CAD build for the part. Positions are in the model's coordinates, mm. Give positions to 0.01 mm unless a question says otherwise; leave off trailing zeros. Order: outer loops, then holes, each group sorted by start corner. A loop starts at its lowest first (then second) coordinate and runs counter-clockwise, first axis right, second up.
```python
from build123d import *

# Parameters (mm, degrees)
SKETCH1_5_R         = 2.5
BOSS_EXTRUDE4_DEPTH = 3


with BuildPart() as part:
    # Sketch1_5 → Boss-Extrude4 (new body)
    # profile 1 of 2: a face of its own
    with BuildSketch(Plane(origin=(0, 0, 0), x_dir=(1, 0, 0), z_dir=(0, 1, 0))):
        Polygon((0, 25.4), (0, 0), (15, 0), (197, 0), (212, 0), (212, 25.4), align=None)
        with Locations(Location((75.666666667, 12.7, 0), (0, 0, 270))):
            Circle(SKETCH1_5_R, mode=Mode.SUBTRACT)
        with Locations(Location((136.333333333, 12.7, 0), (0, 0, 270))):
            Circle(SKETCH1_5_R, mode=Mode.SUBTRACT)
    # profile 2 of 2: a face of its own
    with BuildSketch(Plane(origin=(0, 0, 0), x_dir=(1, 0, 0), z_dir=(0, 1, 0))):
        Polygon((0, -93), (0, 0), (15, 0), (15, -78), (197, -78), (197, 0), (212, 0), (212, -93), align=None)
        with Locations(Location((136.333333333, -85.5, 0), (0, 0, 270))):
            Circle(SKETCH1_5_R, mode=Mode.SUBTRACT)
        with Locations(Location((75.666666667, -85.5, 0), (0, 0, 270))):
            Circle(SKETCH1_5_R, mode=Mode.SUBTRACT)
        with Locations(Location((204.5, -39, 0), (0, 0, 270))):
            Circle(SKETCH1_5_R, mode=Mode.SUBTRACT)
        with Locations(Location((7.5, -39, 0), (0, 0, 270))):
            Circle(SKETCH1_5_R, mode=Mode.SUBTRACT)
    extrude(amount=BOSS_EXTRUDE4_DEPTH)


solid = part.part
```
Item 1: Slice it at B-B (x = 91). Give the cut face in (y, z), and give its area (3 significant figures).
Item 2: Slice it at D-D (y = 0.45). Give the cut face in (x, z), and give its area (3 significant figures).
Item 3: Drop a flat-ended pin along its axis: pin 1 Ø4.5 at (x, z) = (136.33, 85.5) entering from +Y. Give the stop position or say it passes through.
Item 4: Two-plate mould, pull along X, no slides. Class faces 1 (the face through (107, 0, -6)), 2 (the face through (206.61, 1.48, 40.34)): released by +X, released by -X, zero draft, split by the parting line, or undercut.
Item 5: Slice it at A-A (z = 43.5). Give the cut face in (x, y).
Item 6: Slice it at C-C (z = 85.5). Give the cut face in (x, y).
Item 7: Wall check: L1, parallel to X at y = 2.1, z = 39; L2, parallel to X at y = 1.4, z = -12.7; L3, parallel to X at y = 1.7, z = 73. Give the ranges that are in metal, low to high.
A:
1. outline: (0, -25.4) - (3, -25.4) - (3, 0) - (0, 0) - close; (0, 78) - (3, 78) - (3, 93) - (0, 93) - close
1. area: 121 mm2
2. outline: (0, -25.4) - (212, -25.4) - (212, 93) - (0, 93) - close; hole circle Ø5 at (7.5, 39); hole (15, 0) - (197, 0) - (197, 78) - (15, 78) - close; hole circle Ø5 at (75.67, -12.7); hole circle Ø5 at (75.67, 85.5); hole circle Ø5 at (136.33, -12.7); hole circle Ø5 at (136.33, 85.5); hole circle Ø5 at (204.5, 39)
2. area: 10,800 mm2
3. pin 1: passes through
4. face 1: zero draft
4. face 2: undercut
5. outline: (0, 0) - (15, 0) - (15, 3) - (0, 3) - close; (197, 0) - (212, 0) - (212, 3) - (197, 3) - close
6. outline: (0, 0) - (73.17, 0) - (73.17, 3) - (0, 3) - close; (78.17, 0) - (133.83, 0) - (133.83, 3) - (78.17, 3) - close; (138.83, 0) - (212, 0) - (212, 3) - (138.83, 3) - close
7. L1: x = 0 to 5, 10 to 15, 197 to 202, 207 to 212
7. L2: x = 0 to 73.17, 78.17 to 133.83, 138.83 to 212
7. L3: x = 0 to 15, 197 to 212
